Geometry check sheet. Reference: the model listing, model coordinates, mm. Face numbers are marked on the shaded views. Coordinates: 2 decimals unless noted, no trailing zeros. Write each loop counter-clockwise with the first axis right and the second up, starting at its lowest first coordinate (ties: lowest second). Pieces come first, ordered by that corner, then holes. Notation, with made-up numbers: M -35.75,-1 L -27.75,-1 A19 ccw -27.75,31 Z; hole C 44.5,0 d7. An arc over 180 degrees is marked long. Write item = value, one per line. Start each with the question number.
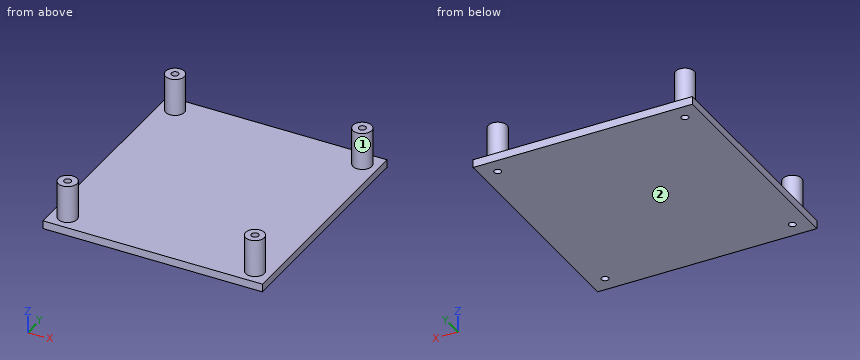
```python
from build123d import *

# Parameters (mm, degrees)
F0_W     = 104.14
F0_H     = 109.982
F1_DEPTH = 3.81
F2_R     = 4.445
F3_DEPTH = 17.78
F6_D     = 3.4


with BuildPart() as f1:
    # F0 (on Top) → F1 (new body)
    with BuildSketch(Plane.XY):
        with Locations((0.4858896136, 8.1733651346)):
            Rectangle(F0_W, F0_H)
    extrude(amount=F1_DEPTH)

    # F2 (on face) → F3 (join)
    with BuildSketch(Plane.XY.offset(3.81)):
        with Locations((-43.9641103864, 55.5443651346)):
            Circle(F2_R)
        with Locations((44.9358896136, 55.5443651346)):
            Circle(F2_R)
        with Locations((-43.9641103864, -39.1976348654)):
            Circle(F2_R)
        with Locations((44.9358896136, -39.1976348654)):
            Circle(F2_R)
    extrude(amount=F3_DEPTH)

    # F6 (through all)
    with Locations(Plane.XY.offset(21.59)):
        with Locations((-43.9641103864, 55.5443651346), (44.9358896136, 55.5443651346), (-43.9641103864, -39.1976348654), (44.9358896136, -39.1976348654)):
            Hole(F6_D / 2)


solid = f1.part
```
Q1. Cross-section at C-C on x = 42. Enter the section's corners in (y, z), and give its area (3 significant figures).
Q2. Cross-section at D-D on y = 47. Enter the section's corners in (x, z), and give its area (3 significant figures).
Q3. Cross-section at A-A on z = 18.5. Enter the section's corners in (x, y) (3 decimals).
Q4. Draft check along Y on the marked faces 1 and 2. Enter one of: pulls with the +Y half, pulls with the -Y half, needs draft (parallel to the pull), parting line crosses it, or undercut.
Q5. Scan lines: L1, parallel to Y at x = 43.5, z = 5; L2, parallel to Y at x = -42.5, z = 1; L3, parallel to Z at x = -8, y = -26.5. Record each from-to range of solid material in increasing order.
Q6. Cross-section at B-B on x = -44. Enter the section's corners in (y, z).
Values found:
q1.outline = M -46.82,0 L 63.16,0 L 63.16,3.81 L 58.88,3.81 L 58.88,21.59 L 52.21,21.59 L 52.21,3.81 L -35.86,3.81 L -35.86,21.59 L -42.54,21.59 L -42.54,3.81 L -46.82,3.81 Z
q1.area = 656 mm²
q2.outline = M -51.58,0 L 52.56,0 L 52.56,3.81 L -51.58,3.81 Z
q2.area = 397 mm²
q3.outline = C -43.964,-39.198 d8.89; C -43.964,55.544 d8.89; C 44.936,-39.198 d8.89; C 44.936,55.544 d8.89; hole C -43.964,-39.198 d3.4; hole C -43.964,55.544 d3.4; hole C 44.936,-39.198 d3.4; hole C 44.936,55.544 d3.4
q4.face_1 = undercut
q4.face_2 = needs draft
q5.L1 = -43.4 to -40.11, -38.29 to -34.99, 51.34 to 54.63, 56.45 to 59.75
q5.L2 = -46.82 to -40.06, -38.33 to 54.68, 56.41 to 63.16
q5.L3 = 0 to 3.81
q6.outline = M -46.82,0 L -40.9,0 L -40.9,21.59 L -43.64,21.59 L -43.64,3.81 L -46.82,3.81 Z; M -37.5,0 L 53.84,0 L 53.84,21.59 L 51.1,21.59 L 51.1,3.81 L -34.75,3.81 L -34.75,21.59 L -37.5,21.59 Z; M 57.24,0 L 63.16,0 L 63.16,3.81 L 59.99,3.81 L 59.99,21.59 L 57.24,21.59 Z
